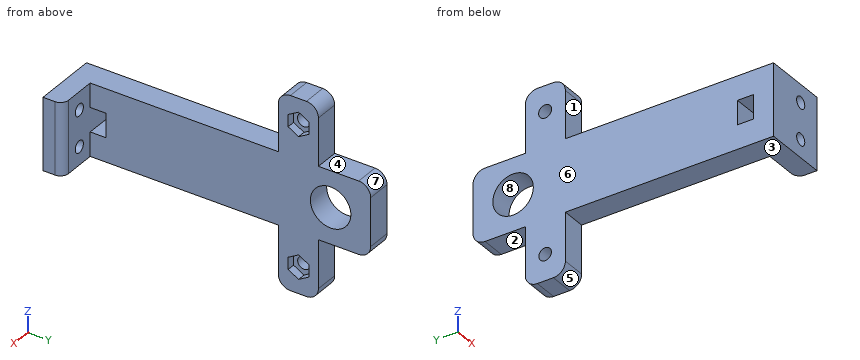
from build123d import *

# Parameters (mm, degrees)
SKETCH1_R                 = 17.45
SKETCH1_R_2               = 12.45
BOSS_EXTRUDE1_DEPTH       = 8
SKETCH2_R                 = 20
SKETCH2_R_2               = 12.45
BOSS_EXTRUDE2_DEPTH       = 2
SKETCH3_R                 = 32.5
SKETCH3_R_2               = 12.45
BOSS_EXTRUDE3_DEPTH       = 4
FILLET1_R                 = 1
BOSS_EXTRUDE6_START       = -4
SKETCH10_W                = 10
SKETCH10_H                = 18
BOSS_EXTRUDE6_DEPTH       = 4
SKETCH4_W                 = 6
SKETCH4_H                 = 18
BOSS_EXTRUDE4_DEPTH       = 75
BOSS_EXTRUDE4_DEPTH_BACK  = 4
SKETCH5_R                 = 5.05
CUT_EXTRUDE1_DEPTH        = 306
CUT_EXTRUDE1_DEPTH_BACK   = 113
SKETCH6_W                 = 6
SKETCH6_H                 = 10
BOSS_EXTRUDE5_DEPTH       = 15
BOSS_EXTRUDE5_DEPTH_BACK  = 32.85
SKETCH7_R                 = 1.629220746
SKETCH7_R_2               = 1.580258945
CUT_EXTRUDE2_DEPTH        = 10
SKETCH9_R                 = 5.05
CUT_EXTRUDE3_DEPTH        = 10
CUT_EXTRUDE3_DEPTH_BACK   = 10
SKETCH11_W                = 9.782596874
SKETCH11_H                = 3.234517514
CUT_EXTRUDE4_DEPTH        = 123
CUT_EXTRUDE4_DEPTH_BACK   = 61
FILLET4_R                 = 3
FILLET5_R                 = 3
SKETCH12_W                = 108.791398151
SKETCH12_H                = 24.041848298
CUT_EXTRUDE5_DEPTH        = 110.678
SKETCH15_R                = 22
CUT_EXTRUDE7_DEPTH        = 4
SKETCH13_R                = 22
SKETCH13_R_2              = 11
SKETCH13_R_3              = 2.75
BOSS_EXTRUDE7_DEPTH       = 4
FILLET6_R                 = 3
CUT_EXTRUDE8_DEPTH        = 5
FILLET7_R                 = 1
BOSS_EXTRUDE8_START       = -3
BOSS_EXTRUDE8_DEPTH       = 9.4
FILLET8_R                 = 3
FILLET8_OF_MIRROR2_R      = 3
CUT_EXTRUDE12_START       = -6
SKETCH21_R                = 6.05
CUT_EXTRUDE12_DEPTH       = 3.8
SKETCH18_W                = 88.746975794
SKETCH18_H                = 20.386854219
CUT_EXTRUDE9_DEPTH        = 10
SKETCH19_W                = 6
SKETCH19_H                = 10.45
BOSS_EXTRUDE9_DEPTH       = 5
FILLET9_R                 = 2
CUT_EXTRUDE13_DEPTH       = 2
SKETCH23_R                = 1
CUT_EXTRUDE14_DEPTH       = 11
CUT_EXTRUDE16_DEPTH       = 1.7
CUT_EXTRUDE17_DEPTH       = 30
CUT_EXTRUDE17_DEPTH_BACK  = 70
SKETCH27_W                = 18
SKETCH27_H                = 5
BOSS_EXTRUDE10_DEPTH      = 10
BOSS_EXTRUDE10_DEPTH_BACK = 6
FILLET10_R                = 2
SKETCH28_W                = 6
SKETCH28_H                = 4
CUT_EXTRUDE18_DEPTH       = 10
SKETCH29_R                = 1.5
CUT_EXTRUDE19_DEPTH       = 100


with BuildPart() as part:
    # Sketch1 → Boss-Extrude1 (new body)
    with BuildSketch(Plane(origin=(0, 0, 0), x_dir=(1, 0, 0), z_dir=(0, 1, 0))):
        Circle(SKETCH1_R)
        Circle(SKETCH1_R_2, mode=Mode.SUBTRACT)
    extrude(amount=BOSS_EXTRUDE1_DEPTH)

    # Sketch2 → Boss-Extrude2 (add)
    with BuildSketch(Plane(origin=(0, 8, 0), x_dir=(1, 0, 0), z_dir=(0, 1, 0))):
        Circle(SKETCH2_R)
        Circle(SKETCH2_R_2, mode=Mode.SUBTRACT)
    extrude(amount=BOSS_EXTRUDE2_DEPTH)

    # Sketch3 → Boss-Extrude3 (add)
    with BuildSketch(Plane(origin=(0, 10, 0), x_dir=(1, 0, 0), z_dir=(0, 1, 0))):
        Circle(SKETCH3_R)
        Circle(SKETCH3_R_2, mode=Mode.SUBTRACT)
    extrude(amount=BOSS_EXTRUDE3_DEPTH)

    # Fillet1
    fillet1_edges = [part.edges().sort_by_distance(p)[0] for p in [
        (-32.5, 14, 0),
    ]]
    fillet(fillet1_edges, radius=FILLET1_R)

    # Sketch10 → Boss-Extrude6 (add)
    with BuildSketch(Plane(origin=(0, 14, 0), x_dir=(1, 0, 0), z_dir=(0, 1, 0)).offset(BOSS_EXTRUDE6_START)):
        with Locations((35.186917696, 0)):
            Rectangle(SKETCH10_W, SKETCH10_H)
        with Locations((-35.186917696, 0)):
            Rectangle(SKETCH10_W, SKETCH10_H)
    extrude(amount=BOSS_EXTRUDE6_DEPTH)

    # Sketch4 → Boss-Extrude4 (add, two sides)
    with BuildSketch(Plane(origin=(0, 14, 0), x_dir=(1, 0, 0), z_dir=(0, 1, 0))) as boss_extrude4_sk:
        with Locations((-37.186917696, 0)):
            Rectangle(SKETCH4_W, SKETCH4_H)
        with Locations((37.186917696, 0)):
            Rectangle(SKETCH4_W, SKETCH4_H)
    extrude(amount=BOSS_EXTRUDE4_DEPTH)
    extrude(boss_extrude4_sk.sketch, amount=-BOSS_EXTRUDE4_DEPTH_BACK)

    # Sketch5 → Cut-Extrude1 (cut, two sides)
    with BuildSketch(Plane.ZY.offset(-34.186917696)) as cut_extrude1_sk:
        with Locations((0, 79)):
            Circle(SKETCH5_R)
    extrude(amount=CUT_EXTRUDE1_DEPTH, mode=Mode.SUBTRACT)
    extrude(cut_extrude1_sk.sketch, amount=-CUT_EXTRUDE1_DEPTH_BACK, mode=Mode.SUBTRACT)

    # Sketch6 → Boss-Extrude5 (add, two sides)
    with BuildSketch(Plane(origin=(0, 0, -9), x_dir=(-1, 0, 0), z_dir=(0, 0, -1))) as boss_extrude5_sk:
        with Locations((37.186917696, 70.95)):
            Rectangle(SKETCH6_W, SKETCH6_H)
    extrude(amount=BOSS_EXTRUDE5_DEPTH)
    extrude(boss_extrude5_sk.sketch, amount=-BOSS_EXTRUDE5_DEPTH_BACK)

    # Sketch7 → Cut-Extrude2 (cut)
    with BuildSketch(Plane(origin=(-34.186917696, 0, 0), x_dir=(0, 0, -1), z_dir=(1, 0, 0))):
        with Locations((-17.5, 71)):
            Circle(SKETCH7_R)
        with Locations((17.5, 71)):
            Circle(SKETCH7_R_2)
    extrude(amount=-CUT_EXTRUDE2_DEPTH, mode=Mode.SUBTRACT)

    # Sketch9 → Cut-Extrude3 (cut, two sides)
    with BuildSketch(Plane(origin=(-34.186917696, 0, 0), x_dir=(0, 0, -1), z_dir=(1, 0, 0))) as cut_extrude3_sk:
        with Locations((0, 79)):
            Circle(SKETCH9_R)
    extrude(amount=CUT_EXTRUDE3_DEPTH, mode=Mode.SUBTRACT)
    extrude(cut_extrude3_sk.sketch, amount=-CUT_EXTRUDE3_DEPTH_BACK, mode=Mode.SUBTRACT)

    # Sketch11 → Cut-Extrude4 (cut, two sides)
    with BuildSketch(Plane.ZY.offset(-34.186917696)) as cut_extrude4_sk:
        with Locations((0, 15.617258757)):
            Rectangle(SKETCH11_W, SKETCH11_H)
    extrude(amount=CUT_EXTRUDE4_DEPTH, mode=Mode.SUBTRACT)
    extrude(cut_extrude4_sk.sketch, amount=-CUT_EXTRUDE4_DEPTH_BACK, mode=Mode.SUBTRACT)

    # Fillet4
    fillet4_edges = [part.edges().sort_by_distance(p)[0] for p in [
        (-37.186917696, 65.95, 23.85),
        (-37.186917696, 75.95, 23.85),
        (-37.186917696, 65.95, -24),
        (-37.186917696, 75.95, -24),
        (-37.186917696, 89, -9),
        (-37.186917696, 89, 9),
    ]]
    fillet(fillet4_edges, radius=FILLET4_R)

    # Fillet5
    fillet5_edges = [part.edges().sort_by_distance(p)[0] for p in [
        (40.186917696, 10, 0),
        (-40.186917696, 10, 0),
    ]]
    fillet(fillet5_edges, radius=FILLET5_R)

    # Sketch12 → Cut-Extrude5 (cut)
    with BuildSketch(Plane(origin=(40.186917696, 0, 0), x_dir=(0, 0, -1), z_dir=(1, 0, 0))):
        with Locations((-12.502918017, -2.020924149)):
            Rectangle(SKETCH12_W, SKETCH12_H)
    extrude(amount=-CUT_EXTRUDE5_DEPTH, mode=Mode.SUBTRACT)

    # Sketch15 → Cut-Extrude7 (cut)
    with BuildSketch(Plane(origin=(0, 14, 0), x_dir=(1, 0, 0), z_dir=(0, 1, 0))):
        Circle(SKETCH15_R)
    extrude(amount=-CUT_EXTRUDE7_DEPTH, mode=Mode.SUBTRACT)

    # Sketch13 → Boss-Extrude7 (add)
    with BuildSketch(Plane(origin=(0, 14, 0), x_dir=(1, 0, 0), z_dir=(0, 1, 0))):
        Circle(SKETCH13_R)
        Circle(SKETCH13_R_2, mode=Mode.SUBTRACT)
        with Locations((0, 17.5)):
            Circle(SKETCH13_R_3, mode=Mode.SUBTRACT)
        with Locations((-15.155444566, -8.75)):
            Circle(SKETCH13_R_3, mode=Mode.SUBTRACT)
        with Locations((15.155444566, -8.75)):
            Circle(SKETCH13_R_3, mode=Mode.SUBTRACT)
    extrude(amount=-BOSS_EXTRUDE7_DEPTH)

    # Fillet6
    fillet6_edges = [part.edges().sort_by_distance(p)[0] for p in [
        (37.186917696, 89, 9),
        (37.186917696, 89, -9),
    ]]
    fillet(fillet6_edges, radius=FILLET6_R)

    # Sketch16 → Cut-Extrude8 (cut)
    with BuildSketch(Plane.XZ.offset(-10)):
        with BuildLine():
            Line((-31.228992939, 9), (-20.29384143, 9))
            ThreePointArc((-20.29384143, 9), (0, 22.2), (20.29384143, 9))
            Line((20.29384143, 9), (31.228992939, 9))
            ThreePointArc((31.228992939, 9), (0, 32.5), (-31.228992939, 9))
        make_face()
    cut_extrude8 = extrude(amount=-CUT_EXTRUDE8_DEPTH, mode=Mode.SUBTRACT)

    # Mirror1: Cut-Extrude8 across plane
    add(cut_extrude8.mirror(Plane.XY), mode=Mode.SUBTRACT)

    # Fillet7
    fillet7_edges = [part.edges().sort_by_distance(p)[0] for p in [
        (0, 14, 22.2),
        (0, 14, -22.2),
    ]]
    fillet(fillet7_edges, radius=FILLET7_R)

    # Sketch17 → Boss-Extrude8 (add)
    with BuildSketch(Plane.XZ.offset(-10).offset(BOSS_EXTRUDE8_START)):
        with BuildLine():
            Line((20.29384143, -9), (40.186917696, -9))
            Line((40.186917696, -9), (40.186917696, 9))
            Line((40.186917696, 9), (20.29384143, 9))
            ThreePointArc((20.29384143, 9), (22.2, 0), (20.29384143, -9))
        make_face()
    boss_extrude8 = extrude(amount=BOSS_EXTRUDE8_DEPTH)

    # Fillet8
    fillet8_edges = [part.edges().sort_by_distance(p)[0] for p in [
        (40.186917696, 3.6, 0),
    ]]
    fillet(fillet8_edges, radius=FILLET8_R)

    # Mirror2: Boss-Extrude8 across plane
    add(boss_extrude8.mirror(Plane(origin=(0, 0, 0), x_dir=(0, 0, 1), z_dir=(1, 0, 0))))

    # Fillet8 of Mirror2
    fillet8_of_mirror2_edges = [part.edges().sort_by_distance(p)[0] for p in [
        (-40.186917696, 3.6, 0),
    ]]
    fillet(fillet8_of_mirror2_edges, radius=FILLET8_OF_MIRROR2_R)

    # Sketch21 → Cut-Extrude12 (cut)
    with BuildSketch(Plane(origin=(40.186917696, 0, 0), x_dir=(0, 0, -1), z_dir=(1, 0, 0)).offset(CUT_EXTRUDE12_START)):
        with Locations((0, 79)):
            Circle(SKETCH21_R)
    extrude(amount=CUT_EXTRUDE12_DEPTH, mode=Mode.SUBTRACT)

    # Sketch18 → Cut-Extrude9 (cut)
    with BuildSketch(Plane(origin=(40.186917696, 0, 0), x_dir=(0, 0, -1), z_dir=(1, 0, 0))):
        with Locations((0, 89.193427109)):
            Rectangle(SKETCH18_W, SKETCH18_H)
    extrude(amount=-CUT_EXTRUDE9_DEPTH, mode=Mode.SUBTRACT)

    # Sketch19 → Boss-Extrude9 (add)
    with BuildSketch(Plane(origin=(0, 79, 0), x_dir=(1, 0, 0), z_dir=(0, 1, 0))):
        with Locations((37.186917696, -11.275)):
            Rectangle(SKETCH19_W, SKETCH19_H)
        with Locations((37.186917696, 11.275)):
            Rectangle(SKETCH19_W, SKETCH19_H)
    extrude(amount=-BOSS_EXTRUDE9_DEPTH)

    # Fillet9
    fillet9_edges = [part.edges().sort_by_distance(p)[0] for p in [
        (37.186917696, 74, 16.5),
        (37.186917696, 74, -16.5),
    ]]
    fillet(fillet9_edges, radius=FILLET9_R)

    # Sketch22 → Cut-Extrude13 (cut)
    with BuildSketch(Plane(origin=(-34.186917696, 0, 0), x_dir=(0, 0, -1), z_dir=(1, 0, 0))):
        Polygon((-15.9988893, 68.4), (-14.4977786, 71), (-15.9988893, 73.6), (-19.0011107, 73.6), (-20.5022214, 71), (-19.0011107, 68.4), align=None)
        Polygon((20.5022214, 71), (19.0011107, 73.6), (15.9988893, 73.6), (14.4977786, 71), (15.9988893, 68.4), (19.0011107, 68.4), align=None)
    extrude(amount=-CUT_EXTRUDE13_DEPTH, mode=Mode.SUBTRACT)

    # Sketch23 → Cut-Extrude14 (cut)
    with BuildSketch(Plane(origin=(0, 79, 0), x_dir=(1, 0, 0), z_dir=(0, 1, 0))):
        with Locations((37.186917696, -12.3)):
            Circle(SKETCH23_R)
        with Locations((37.186917696, 12.3)):
            Circle(SKETCH23_R)
    extrude(amount=-CUT_EXTRUDE14_DEPTH, mode=Mode.SUBTRACT)

    # Sketch24 → Cut-Extrude16 (cut)
    with BuildSketch(Plane.XZ.offset(-74)):
        Polygon((37.186917696, 9.990598923), (39.186917696, 11.145299462), (39.186917696, 13.454700538), (37.186917696, 14.609401077), (35.186917696, 13.454700538), (35.186917696, 11.145299462), align=None)
        Polygon((37.186917696, -14.609401077), (39.186917696, -13.454700538), (39.186917696, -11.145299462), (37.186917696, -9.990598923), (35.186917696, -11.145299462), (35.186917696, -13.454700538), align=None)
    extrude(amount=-CUT_EXTRUDE16_DEPTH, mode=Mode.SUBTRACT)

    # Sketch26 → Cut-Extrude17 (cut, two sides)
    with BuildSketch(Plane(origin=(0, 0, -9), x_dir=(-1, 0, 0), z_dir=(0, 0, -1))) as cut_extrude17_sk:
        Polygon((34.186917696, 14), (34.186917696, 94.491380316), (-54.251567272, 94.491380316), (-54.251567272, -8.918618382), (55.508733715, -8.918618382), (55.508733715, 14), align=None)
    extrude(amount=CUT_EXTRUDE17_DEPTH, mode=Mode.SUBTRACT)
    extrude(cut_extrude17_sk.sketch, amount=-CUT_EXTRUDE17_DEPTH_BACK, mode=Mode.SUBTRACT)

    # Sketch27 → Boss-Extrude10 (add, two sides)
    with BuildSketch(Plane(origin=(-34.186917696, 0, 0), x_dir=(0, 0, -1), z_dir=(1, 0, 0))) as boss_extrude10_sk:
        with Locations((0, 16.5)):
            Rectangle(SKETCH27_W, SKETCH27_H)
    extrude(amount=BOSS_EXTRUDE10_DEPTH)
    extrude(boss_extrude10_sk.sketch, amount=-BOSS_EXTRUDE10_DEPTH_BACK)

    # Fillet10
    fillet10_edges = [part.edges().sort_by_distance(p)[0] for p in [
        (-24.186917696, 19, 0),
    ]]
    fillet(fillet10_edges, radius=FILLET10_R)

    # Sketch28 → Cut-Extrude18 (cut)
    with BuildSketch(Plane(origin=(-34.186917696, 0, 0), x_dir=(0, 0, -1), z_dir=(1, 0, 0))):
        with Locations((0, 21)):
            Rectangle(SKETCH28_W, SKETCH28_H)
    extrude(amount=-CUT_EXTRUDE18_DEPTH, mode=Mode.SUBTRACT)

    # Sketch29 → Cut-Extrude19 (cut)
    with BuildSketch(Plane(origin=(0, 19, 0), x_dir=(1, 0, 0), z_dir=(0, 1, 0))):
        with Locations((-30.186917696, -4.5)):
            Circle(SKETCH29_R)
        with Locations((-30.186917696, 4.5)):
            Circle(SKETCH29_R)
    extrude(amount=-CUT_EXTRUDE19_DEPTH, mode=Mode.SUBTRACT)


solid = part.part
Read the model definition and answer for the solid it produces. Units are mm, in the model's axes. Face numbers are marked on the shaded views. A direction names the side the tool comes from. Give positions to 0.01 mm unless a question says otherwise; leave off trailing zeros. Write each loop counter-clockwise with the first axis right and the second up, starting at its lowest first coordinate (ties: lowest second). Pieces come first, ordered by that corner, then holes. Notation, with made-up numbers: (50, 24) -> (71, 24) arc R22 ccw to (71, 42) -> close; hole circle Ø4 at (-33.75, -7). An arc over 180 degrees is marked (long way). Answer as a JSON object with one key per item and string values. Group by question number.
1) Each of these flat-tipped pins is pushed along its axis until it touches: P1, Ø1.6, axis at x = -35, z = -17.5, coming from the +Y side; P2, Ø1, axis at x = -35, z = 18, coming from the -Y side; P3, Ø8, axis at x = -32, y = 62.5, coming from the +Z side. Where does it stop, or does it pass through?
2) Find section B-B (x = -38.5). Write down the section's boundary in (y, z).
3) Find section D-D (y = 77). Write down the section's boundary in (x, z), and give its area (3 significant figures).
4) Find section A-A (z = -17.5). Write down the section's boundary in (x, y).
5) A tool of negligible diameter and unlimited length cuts with its end or side. For the marked faces 1, 2, 3 and 4, from which of +Z, -Z, +X, -X, +Y, -Y can it reach the whole face along a straight path? Write none if from no direction.
6) Consider L1, parallel to Y at x = -36.35, z = 0; L2, parallel to Z at x = -37.9, y = 71; L3, parallel to Y at x = -37.85, z = 17.5. Determine where each line is inside the solid, lowest interval first. Write a range as from..to.
7) The mould has two halves that part along Y. Classify the marked faces 5, 6, 7 and 8: +Y half, -Y half, draft (parallel to the pull), parting line (faces both ways), or undercut.
8) Find section C-C (z = 0). Write down the section's boundary in (x, y), and give its area (3 significant figures).
Values follow:
{
 "1": {"P1": "stops at y = 75.95", "P2": "stops at y = 65.95", "P3": "stops at z = 9"},
 "2": {"outline": "(14, -9) -> (65.95, -9) -> (65.95, -21) arc R3 ccw to (68.95, -24) -> (72.95, -24) arc R3 ccw to (75.95, -21) -> (75.95, -9) -> (86, -9) arc R3 ccw to (89, -6) -> (89, 6) arc R3 ccw to (86, 9) -> (75.95, 9) -> (75.95, 20.85) arc R3 ccw to (72.95, 23.85) -> (68.95, 23.85) arc R3 ccw to (65.95, 20.85) -> (65.95, 9) -> (14, 9) -> close; hole (19, -3) -> (23, -3) -> (23, 3) -> (19, 3) -> close; hole circle Ø3.26 at (71, 17.5); hole circle Ø3.16 at (71, -17.5); hole circle Ø10.1 at (79, 0)"},
 "3": {"outline": "(-40.19, -9) -> (-34.19, -9) -> (-34.19, -4.64) -> (-40.19, -4.64) -> close; (-40.19, 4.64) -> (-34.19, 4.64) -> (-34.19, 9) -> (-40.19, 9) -> close", "area": "52.4 mm2"},
 "4": {"outline": "(-40.19, 65.95) -> (-34.19, 65.95) -> (-34.19, 68.4) -> (-36.19, 68.4) -> (-36.19, 69.42) -> (-40.19, 69.42) -> close; (-40.19, 72.58) -> (-36.19, 72.58) -> (-36.19, 73.6) -> (-34.19, 73.6) -> (-34.19, 75.95) -> (-40.19, 75.95) -> close"},
 "5": {"face 1": "+Z, +X, -X, -Y", "face 2": "-Z, +X, -X, +Y", "face 3": "-Z, +X, -X, -Y", "face 4": "+Z, +X, -X, +Y"},
 "6": {"L1": "y = 14..19, 23..73.95, 84.05..89", "L2": "z = -24..-19.08, -15.92..15.87, 19.13..23.85", "L3": "y = 65.95..69.37, 72.63..75.95"},
 "7": {"face 5": "-Y half", "face 6": "draft", "face 7": "+Y half", "face 8": "undercut"},
 "8": {"outline": "(-40.19, 14) -> (-24.19, 14) -> (-24.19, 17) arc R2 ccw to (-26.19, 19) -> (-40.19, 19) -> close; (-40.19, 23) -> (-34.19, 23) -> (-34.19, 73.95) -> (-40.19, 73.95) -> close; (-40.19, 84.05) -> (-34.19, 84.05) -> (-34.19, 89) -> (-40.19, 89) -> close", "area": "415 mm2"}
}
